Here's how the part is built. I have some questions about the finished solid (model axes, mm). A direction names the side the tool comes from. Round coordinates to 2 decimals unless told otherwise and drop trailing zeros. Loops run counter-clockwise (first coordinate to the right, second up) from the corner with the lowest first, then second, coordinate; pieces in that order, holes last. Notation, with made-up numbers: (-6.5, -32) - (29.5, -32) arc R14 ccw to (29.5, -5) - close; hole circle Ø3 at (2.5, -23). An arc over 180 degrees is marked (long way). Answer as a JSON object with one key per item and string values. Group by question number.
1) I want a section at A-A, the plane z = 0.75. Please give me the cut outline in (x, y), then the cut area to 3 significant figures.
2) Which directions (+Z, -Z, +X, -X, +Y, -Y) give clear straight access to the entire face, cutting with the end or side of a thin tool? Please do faces 4 (the face through (-2.167, -3.725, 3.944)), 5 (the face through (-4, 4, 0)).
3) If I drill on line 1 along Y through (x, z) = (0, 0.5); line 2 along X through (y, z) = (-2, 1.75); line 3 along X through (y, z) = (3, 1.5), over which ranges is the centre line in solid material (lowest first)? Write a range as [from, to].
4) Will these pins go through, and if not, where does the flat tip stop? P1, Ø3, axis at x = 11.5, z = 4.5, coming from the +Y side; P2, Ø1.5, axis at x = -2.5, y = -7.5, coming from the +Z side; P3, Ø3, axis at x = 3, z = 3, coming from the +Y side.
5) I want a section at B-B, the plane x = 0. Please give me the cut outline in (y, z), then the cut area to 3 significant figures.
6) I want a section at C-C, the plane z = 2.75. Please give me the cut outline in (x, y), then the cut area to 3 significant figures.
7) If we mould it in two halves opening along Y, with no side actions, what happens to faces 1 (the face through (-1.596, 7.188, 7.845)), 2 (the face through (0, 5, 8)), 3 (the face through (-2.14, 3.74, 3.94))? For each: pulls with the +Y half, pulls with the -Y half, needs draft (parallel to the pull), parting line crosses it, or undercut.
from build123d import *

# Parameters (mm, degrees)
F3_DEPTH = 25
F4_R     = 2


with BuildPart() as f1:
    # F0 (on Front) → F1 (revolve)
    with BuildSketch(Plane.XZ):
        with BuildLine():
            Line((0, 8), (0, 0))
            Line((0, 0), (17.5, 0))
            Line((17.5, 0), (17.5, 0.203019))
            ThreePointArc((17.5, 0.203019), (16.674205, 2.955474), (14.469596, 4.798744))
            Line((14.469596, 4.798744), (7, 8))
            Line((7, 8), (0, 8))
        make_face()
    revolve(axis=Axis((0, 0, -4.491808), (0, 0, -1)))

    # F2 (on face) → F3 (cut)
    with BuildSketch(Plane.XY.offset(8)):
        Polygon((2.309401, 4), (-2.309401, 4), (-4.618802, 0), (-2.309401, -4), (2.309401, -4), (4.618802, 0), align=None)
    extrude(amount=-F3_DEPTH, mode=Mode.SUBTRACT)

    # F4
    f4_edges = [f1.edges().sort_by_distance(p)[0] for p in [
        (-2.309401, 4, 4),
        (-4.618802, 0, 4),
        (2.309401, 4, 4),
        (4.618802, 0, 4),
        (-2.309401, -4, 4),
        (2.309401, -4, 4),
    ]]
    fillet(f4_edges, radius=F4_R)


solid = f1.part
Outcome:
{
 "1": {"outline": "circle Ø34.94 at (0, 0); hole (-4.04, -1) - (-2.89, -3) arc R2 ccw to (-1.15, -4) - (1.15, -4) arc R2 ccw to (2.89, -3) - (4.04, -1) arc R2 ccw to (4.04, 1) - (2.89, 3) arc R2 ccw to (1.15, 4) - (-1.15, 4) arc R2 ccw to (-2.89, 3) - (-4.04, 1) arc R2 ccw to start", "area": "905 mm^2"},
 "2": {"face 4": "+Z, -Z", "face 5": "-Z, +X, -X, +Y, -Y"},
 "3": {"line 1": "[-17.49, -4], [4, 17.49]", "line 2": "[-17.14, -3.46], [3.46, 17.14]", "line 3": "[-17.07, -2.89], [2.89, 17.07]"},
 "4": {"P1": "y = 12.55", "P2": "z = 7.93", "P3": "y = 17.13"},
 "5": {"outline": "(-17.5, 0) - (-4, 0) - (-4, 8) - (-7, 8) - (-14.47, 4.8) arc R5 ccw to (-17.5, 0.2) - close; (4, 0) - (17.5, 0) - (17.5, 0.2) arc R5 ccw to (14.47, 4.8) - (7, 8) - (4, 8) - close", "area": "165 mm^2"},
 "6": {"outline": "circle Ø33.61 at (0, 0); hole (-4.04, -1) - (-2.89, -3) arc R2 ccw to (-1.15, -4) - (1.15, -4) arc R2 ccw to (2.89, -3) - (4.04, -1) arc R2 ccw to (4.04, 1) - (2.89, 3) arc R2 ccw to (1.15, 4) - (-1.15, 4) arc R2 ccw to (-2.89, 3) - (-4.04, 1) arc R2 ccw to start", "area": "833 mm^2"},
 "7": {"face 1": "parting line crosses it", "face 2": "needs draft", "face 3": "undercut"}
}
